Here's the drawing with two shaded views (mm, measured from the low corner). I have some questions. A direction names the side the tool comes from. Coordinates: 2 decimals unless noted, no trailing zeros. Write each loop counter-clockwise with the first axis right and the second up, starting at its lowest first coordinate (ties: lowest second). Pieces come first, ordered by that corner, then holes. Notation, with made-up numbers: (80, 60) - (91, 60) arc R12 ccw to (91, 82) - close; hole circle Ø8 at (-30.5, -7). An arc over 180 degrees is marked (long way). Answer in a Markdown table with one row per item. Add a question column.
Item 1: Which directions (+Z, -Z, +X, -X, +Y, -Y) give clear straight access to the entire face, cutting with the end or side of a thin tool? Please do the marked faces 4 and 5.
Item 2: Imagine slicing it at D-D (x = 50). Please give me the cut outline in (y, z).
Item 3: Imagine slicing it at A-A (y = 12.5). Please give me the cut outline in (x, z).
Item 4: We'd pull the mould along Z, two halves only. Please class the marked faces 1, 2 and 3: +Z half, -Z half, draft (parallel to the pull), parting line (faces both ways), or undercut.
Item 5: I'm going to push flat-ended pins straight in: pin 1 (4 mm diameter, centred on x = 55, z = 3, fed in from +Y); pin 2 (2.5 mm diameter, centred on y = 58.5, z = 1.5, fed in from -X); pin 3 (2.5 mm diameter, centred on x = 51, z = 175, fed in from -Y). Where does each tip first touch, or does it pass through?
Item 6: Imagine slicing it at C-C (y = 91). Please give me the cut outline in (x, z).
Item 7: If I drill on probe 1 along Y at (x, z) = (91.25, 2.65); probe 2 along Z at (x, y) = (93.5, 38); probe 3 along Y at (x, z) = (12.5, 173.1), over which ranges is the centre line in solid material (lowest first)? Write a range as from..to.
Item 8: Imagine slicing it at B-B (x = 91.25). Please give me the cut outline in (y, z).
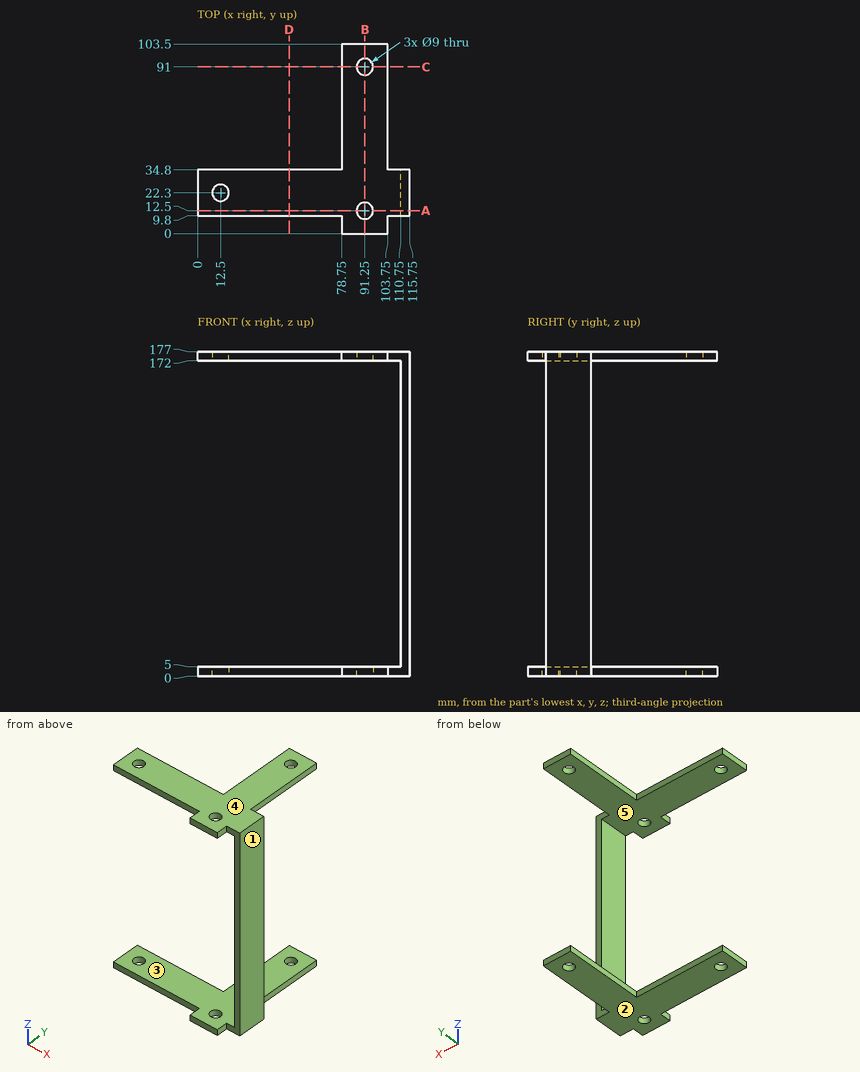
Here are the results:
| question | item | result |
|---|---|---|
| 1 | face 4 | +Z, +X, -X, +Y, -Y |
| 1 | face 5 | -X, +Y, -Y |
| 2 | outline | (9.8, 0) - (34.8, 0) - (34.8, 5) - (9.8, 5) - close; (9.8, 172) - (34.8, 172) - (34.8, 177) - (9.8, 177) - close |
| 3 | outline | (0, 0) - (86.75, 0) - (86.75, 5) - (0, 5) - close; (0, 172) - (86.75, 172) - (86.75, 177) - (0, 177) - close; (95.75, 0) - (115.75, 0) - (115.75, 177) - (95.75, 177) - (95.75, 172) - (110.75, 172) - (110.75, 5) - (95.75, 5) - close |
| 4 | face 1 | draft |
| 4 | face 2 | -Z half |
| 4 | face 3 | undercut |
| 5 | pin 1 | stops at y = 34.8 |
| 5 | pin 2 | stops at x = 78.75 |
| 5 | pin 3 | stops at y = 9.8 |
| 6 | outline | (78.75, 0) - (86.75, 0) - (86.75, 5) - (78.75, 5) - close; (78.75, 172) - (86.75, 172) - (86.75, 177) - (78.75, 177) - close; (95.75, 0) - (103.75, 0) - (103.75, 5) - (95.75, 5) - close; (95.75, 172) - (103.75, 172) - (103.75, 177) - (95.75, 177) - close |
| 7 | probe 1 | y = 0..8, 17..86.5, 95.5..103.5 |
| 7 | probe 2 | z = 0..5, 172..177 |
| 7 | probe 3 | y = 9.8..17.8, 26.8..34.8 |
| 8 | outline | (0, 0) - (8, 0) - (8, 5) - (0, 5) - close; (0, 172) - (8, 172) - (8, 177) - (0, 177) - close; (17, 0) - (86.5, 0) - (86.5, 5) - (17, 5) - close; (17, 172) - (86.5, 172) - (86.5, 177) - (17, 177) - close; (95.5, 0) - (103.5, 0) - (103.5, 5) - (95.5, 5) - close; (95.5, 172) - (103.5, 172) - (103.5, 177) - (95.5, 177) - close |
